Build history of the part. All positions in model axes, mm. Face numbers are marked on the shaded views. A direction names the side the tool comes from. Give positions to 0.01 mm unless a question says otherwise; leave off trailing zeros. Order: outer loops, then holes, each group sorted by start corner. A loop starts at its lowest first (then second) coordinate and runs counter-clockwise, first axis right, second up. Notation, with made-up numbers: (21.5, -7) - (56.5, -7) arc R17 ccw to (56.5, 2) - close; hole circle Ø5 at (23, 18.5). An arc over 180 degrees is marked (long way). Write each question's results on one line, items separated by ' | '. Start each with the question number.
1) Cut at D-D on z = -6.5. List the corners of the cut face in (x, y) (3 decimals), plus the area to 3 significant figures.
2) Cut at B-B on z = -10.5. List the corners of the cut face in (x, y) (3 decimals), plus the area to 3 significant figures.
3) Two-plate mould, pull along Z, no slides. Class the marked faces 3, 4 and 5: +Z half, -Z half, draft (parallel to the pull), parting line (faces both ways), or undercut.
4) Drop flat-ended pins along their axis: pin 1 Ø5 at (x, z) = (-7.5, 13) entering from -Y; pin 2 Ø0.6 at (x, z) = (15.5, 1) entering from +Y; pin 3 Ø4 at (x, z) = (11, -1) entering from -Y; pin 4 Ø1.5 at (x, z) = (0.5, -5.5) entering from +Y. Give the stop position or say it passes through.
5) Cut at C-C on x = 0. List the corners of the cut face in (y, z), plus the area to 3 significant figures.
6) Drill centre lines: line 1 along X through (y, z) = (13, 4) (3 decimals); line 2 along Z through (x, y) = (-8.5, -0.5); line 3 along Z through (x, y) = (1, -5.5). Where is each one in solid material? Low to high. Write a range as from..to.
7) Tool access for the marked faces 1 and 2: list every direction of +Z, -Z, +X, -X, +Y, -Y with a clear straight run to the whole face (end or side of a thin tool).
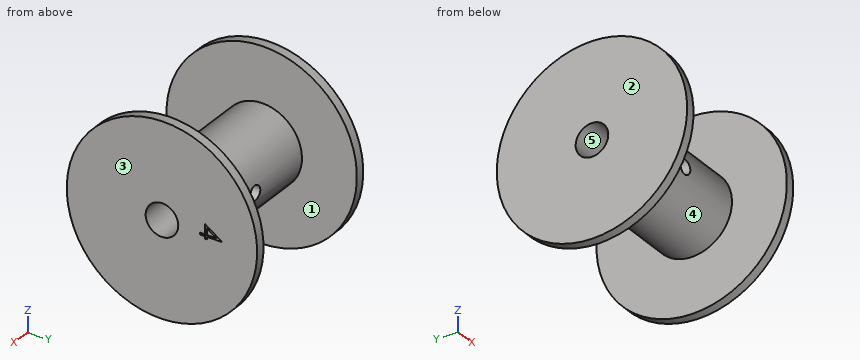
from build123d import *

# Parameters (mm, degrees)
SKETCH1_W               = 13.97
SKETCH1_H               = 4.8006
CUT_EXTRUDE1_DEPTH      = 32.270123521
CUT_EXTRUDE1_DEPTH_BACK = 32.270123521
SKETCH2_R               = 1.5
CUT_EXTRUDE2_DEPTH      = 1.27


with BuildPart() as part:
    # Sketch1 → Revolve1 (revolve)
    with BuildSketch(Plane.XY, mode=Mode.PRIVATE) as revolve1_sk:
        with Locations((6.985, 5.6642)):
            Rectangle(SKETCH1_W, SKETCH1_H)
        Polygon((13.97, 8.0645), (13.97, 3.2639), (15.875, 3.2639), (15.875, 19.05), (13.97, 19.05), align=None)
        with Locations((-6.985, 5.6642)):
            Rectangle(SKETCH1_W, SKETCH1_H)
        Polygon((-15.875, 3.2639), (-13.97, 3.2639), (-13.97, 8.0645), (-13.97, 19.05), (-15.875, 19.05), align=None)
    revolve(revolve1_sk.sketch.rotate(Axis((-15.275524476, 0, 0), (1, 0, 0)), 90), axis=Axis((-15.275524476, 0, 0), (1, 0, 0)))

    # Sketch2 → Cut-Extrude1 (cut, two sides: drawn at the far end of the back side and taken through both)
    with BuildSketch(Plane(origin=(0, 0, 0), x_dir=(1, 0, 0), z_dir=(0, 1, 0)).offset(-CUT_EXTRUDE1_DEPTH_BACK)):
        with Locations(Location((0, 0, 0), (0, 0, 90))):
            Circle(SKETCH2_R)
    extrude(amount=CUT_EXTRUDE1_DEPTH + CUT_EXTRUDE1_DEPTH_BACK, mode=Mode.SUBTRACT)

    # Sketch3 → Cut-Extrude2 (cut)
    with BuildSketch(Plane(origin=(15.875, 0, 0), x_dir=(0, 0, -1), z_dir=(1, 0, 0))):
        Polygon((0.253501878, 11.957106949), (0.330672017, 11.957106949), (0.330672017, 9.026337718), (0.819133555, 9.026337718), (0.819133555, 8.592149684), (0.330672017, 8.592149684), (0.330672017, 7.615226607), (-0.049242513, 7.615226607), (-0.049242513, 8.592149684), (-2.057362172, 8.592149684), align=None)
        Polygon((-0.049242513, 9.026337718), (-0.049242513, 10.863156629), (-1.310253464, 9.026337718), align=None, mode=Mode.SUBTRACT)
    extrude(amount=-CUT_EXTRUDE2_DEPTH, mode=Mode.SUBTRACT)


solid = part.part
Results:
1) outline: (-15.875, -17.907) - (-13.97, -17.907) - (-13.97, -4.773) - (13.97, -4.773) - (13.97, -17.907) - (15.875, -17.907) - (15.875, 17.907) - (13.97, 17.907) - (13.97, 4.773) - (-13.97, 4.773) - (-13.97, 17.907) - (-15.875, 17.907) - close | area: 403 mm^2
2) outline: (-15.875, -15.895) - (-13.97, -15.895) - (-13.97, 15.895) - (-15.875, 15.895) - close; (13.97, -15.895) - (15.875, -15.895) - (15.875, 15.895) - (13.97, 15.895) - close | area: 121 mm^2
3) face 3: draft | face 4: parting line | face 5: undercut
4) pin 1: through | pin 2: y = 19.04 | pin 3: y = -8.06 | pin 4: y = 6.52
5) outline: (-7.92, -1.5) arc R8.06 ccw to (7.92, -1.5) - (2.9, -1.5) arc R3.26 cw to (-2.9, -1.5) - close; (-7.92, 1.5) - (-2.9, 1.5) arc R3.26 cw to (2.9, 1.5) - (7.92, 1.5) arc R8.06 ccw to start | area: 142 mm^2
6) line 1: -15.875..-13.97, 13.97..15.875 | line 2: -8.05..-3.23, 3.23..8.05 | line 3: -5.9..-1.12, 1.12..5.9
7) face 1: none | face 2: +Z, -Z, -X, +Y, -Y
